from build123d import *

# Parameters (mm, degrees)
F0_R     = 3.175
F1_DEPTH = 3.048


with BuildPart() as f1:
    # F0 (on Front) → F1 (new body)
    with BuildSketch(Plane.XZ):
        with BuildLine():
            ThreePointArc((9.525, 0), (6.7351920908, 6.7351920908), (0, 9.525))
            ThreePointArc((0, 9.525), (-6.4912990883, 6.9705567315), (-9.500885786, 0.6773435479))
            Line((-9.500885786, 0.6773435479), (-9.525, 0))
            ThreePointArc((-9.525, 0), (-6.7351920908, -6.7351920908), (0, -9.525))
            ThreePointArc((0, -9.525), (6.7351920908, -6.7351920908), (9.525, 0))
        make_face()
        with BuildLine():
            ThreePointArc((3.175, 0), (-2.2450640303, -2.2450640303), (0, 3.175))
            ThreePointArc((0, 3.175), (2.2450640303, 2.2450640303), (3.175, 0))
        make_face(mode=Mode.SUBTRACT)
        with BuildLine():
            ThreePointArc((-9.500885786, 0.6773435479), (-6.4912990883, 6.9705567315), (0, 9.525))
            Line((0, 9.525), (0, 36.5125))
            ThreePointArc((0, 36.5125), (-5.7116327839, 38.9380895153), (-7.9324746146, 44.7324052746))
            Line((-7.9324746146, 44.7324052746), (-9.500885786, 0.6773435479))
        make_face()
        with BuildLine():
            Line((0, 36.5125), (0, 9.525))
            ThreePointArc((0, 9.525), (6.7351920908, 6.7351920908), (9.525, 0))
            ThreePointArc((9.525, 0), (6.7351920908, -6.7351920908), (0, -9.525))
            Line((0, -9.525), (61.9003804205, -15.7942028036))
            ThreePointArc((61.9003804205, -15.7942028036), (47.6334382359, 0.5175353004), (62.9330357143, 15.8648724073))
            Line((62.9330357143, 15.8648724073), (16.9780821582, 14.2225763491))
            ThreePointArc((16.9780821582, 14.2225763491), (11.2768653549, 16.3488776236), (8.7490183423, 21.8837687364))
            Line((8.7490183423, 21.8837687364), (7.9324362036, 44.7334821429))
            ThreePointArc((7.9324362036, 44.7334821429), (7.9362339499, 44.5917636831), (7.9375, 44.45))
            ThreePointArc((7.9375, 44.45), (5.6126600757, 38.8373399243), (0, 36.5125))
        make_face()
        with BuildLine():
            ThreePointArc((-7.9324746146, 44.7324052746), (-5.7116327839, 38.9380895153), (0, 36.5125))
            ThreePointArc((0, 36.5125), (5.6126600757, 38.8373399243), (7.9375, 44.45))
            ThreePointArc((7.9375, 44.45), (7.9362339499, 44.5917636831), (7.9324362036, 44.7334821429))
            ThreePointArc((7.9324362036, 44.7334821429), (-0.0005387766, 52.3874999817), (-7.9324746146, 44.7324052746))
        make_face()
        with BuildLine():
            ThreePointArc((3.175, 44.45), (2.2450640303, 42.2049359697), (0, 41.275))
            ThreePointArc((0, 41.275), (-2.2450640303, 46.6950640303), (3.175, 44.45))
        make_face(mode=Mode.SUBTRACT)
        with BuildLine():
            Line((-9.525, 0), (-9.500885786, 0.6773435479))
            ThreePointArc((-9.500885786, 0.6773435479), (-9.5189695375, 0.3388863295), (-9.525, 0))
        make_face()
        with BuildLine():
            ThreePointArc((62.9330357143, 15.8648724073), (47.6334382359, 0.5175353004), (61.9003804205, -15.7942028036))
            ThreePointArc((61.9003804205, -15.7942028036), (63.6936154008, -15.8738192656), (65.484375, -15.7504882737))
            ThreePointArc((65.484375, -15.7504882737), (75.40625, -10.5003255158), (79.375, 0))
            ThreePointArc((79.375, 0), (75.40625, 10.5003255158), (65.484375, 15.7504882737))
            ThreePointArc((65.484375, 15.7504882737), (64.2110092937, 15.8590696696), (62.9330357143, 15.8648724073))
        make_face()
        with Locations((63.5, 0)):
            Circle(F0_R, mode=Mode.SUBTRACT)
        with BuildLine():
            ThreePointArc((79.375, 0), (75.40625, -10.5003255158), (65.484375, -15.7504882737))
            Line((65.484375, -15.7504882737), (115.490625, -9.4502929642))
            ThreePointArc((115.490625, -9.4502929642), (104.775, 0), (115.490625, 9.4502929642))
            Line((115.490625, 9.4502929642), (65.484375, 15.7504882737))
            ThreePointArc((65.484375, 15.7504882737), (75.40625, 10.5003255158), (79.375, 0))
        make_face()
        with Locations((100.0252, -3.175)):
            Circle(F0_R, mode=Mode.SUBTRACT)
        with BuildLine():
            ThreePointArc((115.490625, 9.4502929642), (104.775, 0), (115.490625, -9.4502929642))
            ThreePointArc((115.490625, -9.4502929642), (121.44375, -6.3001953095), (123.825, 0))
            ThreePointArc((123.825, 0), (121.44375, 6.3001953095), (115.490625, 9.4502929642))
        make_face()
        with Locations((114.3, 0)):
            Circle(F0_R, mode=Mode.SUBTRACT)
    extrude(amount=F1_DEPTH)


solid = f1.part
Input: part model. Units: mm. Frame: model coordinates. A direction names the side the tool comes from. Give positions to 0.01 mm unless a question says otherwise; leave off trailing zeros. Order: outer loops, then holes, each group sorted by start corner. A loop starts at its lowest first (then second) coordinate and runs counter-clockwise, first axis right, second up. Notation, with made-up numbers: M 64,58.25 L 122,58.25 A15 ccw 122,86.25 Z; hole C -3,18.25 d1. An arc over 180 degrees is marked long. Answer as a JSON object with one key per item and string values.
1. Reachability of faces 4 (the cylindrical face through (11.34, -1.5, 16.29)), 5 (the flat face through (41, 0, 4)) from +Z, -Z, +X, -X, +Y, -Y: full face, straight path, thin tool, end or side. Return the list, or none.
Result sheet:
{"face 4": "+Z, +Y, -Y", "face 5": "+Z, -Z, +X, -X, +Y"}
2. Cut plane C-C, the plane z = 36.5. Output: boundary loops of the cut face in (x, y).
Result sheet:
{"outline": "M -8.23,-3.05 L 8.23,-3.05 L 8.23,0 L -8.23,0 Z"}
3. Pull-direction query (Z, two-part tool) for faces 1 (the cylindrical face through (0.17, -1.503, 52.386)), 2 (the cylindrical face through (63.668, -1.503, -15.874)), 3 (the cylindrical face through (117.33, -1.5, 0.95)); classes: +Z half, -Z half, draft (parallel to the pull), parting line (faces both ways), or undercut.
Result sheet:
{"face 1": "+Z half", "face 2": "-Z half", "face 3": "undercut"}
4. Cut plane A-A, the plane y = -1.05. State how many separate pieces and enclosed holes the cut face has, and give its area (3 significant figures).
Result sheet:
{"separate pieces": "1", "enclosed holes": "5", "area": "3,860 mm²"}
5. Ray query, line 1 (Z direction, x = 0, y = -1.6) (1 decimal); line 2 (X direction, y = -1.4, z = 44.45) (3 decimals); line 3 (Z direction, x = 63.5, y = -0.65) (3 decimals). Return the intervals inside material, ascending. Write a range as [from, to].
Result sheet:
{"line 1": "[-9.5, -3.2], [3.2, 41.3], [47.6, 52.4]", "line 2": "[-7.943, -3.175], [3.175, 7.943]", "line 3": "[-15.875, -3.175], [3.175, 15.875]"}
6. Cut plane B-B, the plane x = 104.5. Output: boundary loops of the cut face in (y, z).
Result sheet:
{"outline": "M -3.05,-10.83 L 0,-10.83 L 0,10.83 L -3.05,10.83 Z"}
